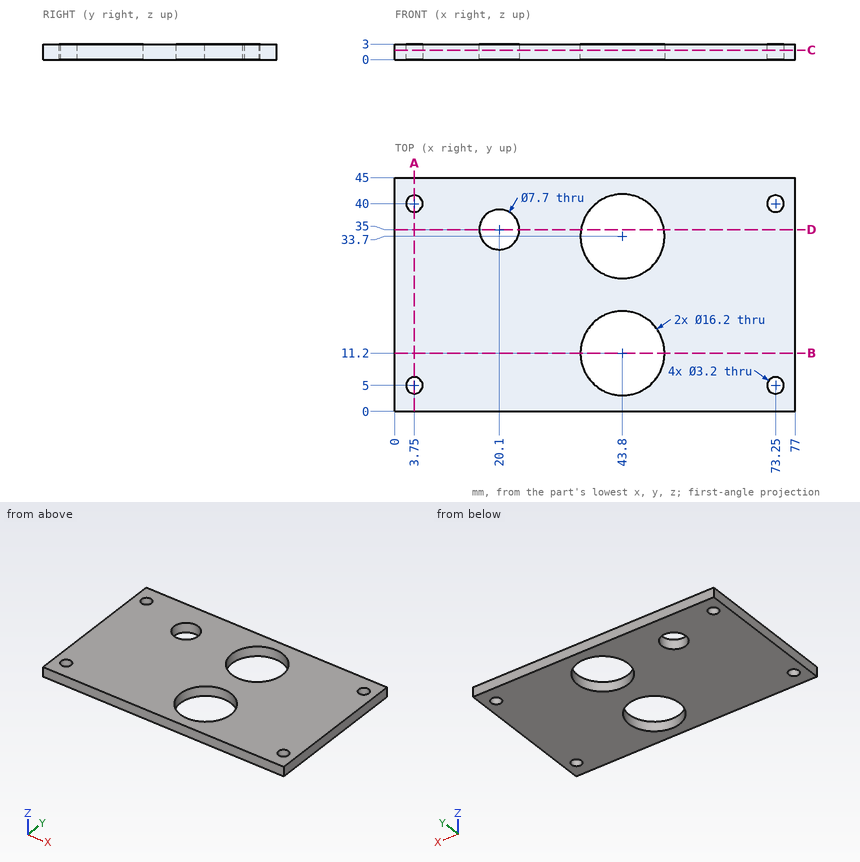
Could you check a few things on this drawing? It's one solid part, dimensions in mm from its lowest x, y, z. Give positions to 0.01 mm unless a question says otherwise; leave off trailing zeros. Order: outer loops, then holes, each group sorted by start corner. A loop starts at its lowest first (then second) coordinate and runs counter-clockwise, first axis right, second up. Notation, with made-up numbers: (46.25, 85.25) -> (93.25, 85.25) arc R24 cw to (93.25, 111.25) -> close; hole circle Ø8 at (-38, 17.25). An arc over 180 degrees is marked (long way). Use CSV: the item, a comma, the result in double quotes. Start each with the question number.
Item 1: I'm going to push a flat-ended pin straight in: P1, Ø1.9, axis at x = 3.75, y = 5, coming from the -Z side. Where does the tip first touch, or does it pass through?
Item 2: Suppose I cut it at A-A (x = 3.75). List the corners of the cut face in (y, z) for me.
Item 3: Suppose I cut it at B-B (y = 11.2). List the corners of the cut face in (x, z) for me, and give its area (3 significant figures).
Item 4: Suppose I cut it at C-C (z = 1.8). List the corners of the cut face in (x, y) for me, and give its area (3 significant figures).
Item 5: If I drill on probe 1 along Y at (x, z) = (43.8, 1.4); probe 2 along Y at (x, z) = (73.25, 2.3); probe 3 along X at (y, z) = (6, 1.5), over which ranges is the centre line in solid material (lowest first)? Write a range as [from, to].
Item 6: Suppose I cut it at D-D (y = 35). List the corners of the cut face in (x, z) for me (3 decimals), and give its area (3 significant figures).
Answer block:
1,P1,"passes through"
2,outline,"(0, 0) -> (3.4, 0) -> (3.4, 3) -> (0, 3) -> close; (6.6, 0) -> (38.4, 0) -> (38.4, 3) -> (6.6, 3) -> close; (41.6, 0) -> (45, 0) -> (45, 3) -> (41.6, 3) -> close"
3,outline,"(0, 0) -> (35.7, 0) -> (35.7, 3) -> (0, 3) -> close; (51.9, 0) -> (77, 0) -> (77, 3) -> (51.9, 3) -> close"
3,area,"182 mm^2"
4,outline,"(0, 0) -> (77, 0) -> (77, 45) -> (0, 45) -> close; hole circle Ø3.2 at (3.75, 5); hole circle Ø3.2 at (3.75, 40); hole circle Ø7.7 at (20.1, 35); hole circle Ø16.2 at (43.8, 11.2); hole circle Ø16.2 at (43.8, 33.7); hole circle Ø3.2 at (73.25, 5); hole circle Ø3.2 at (73.25, 40)"
4,area,"2,970 mm^2"
5,probe 1,"y = [0, 3.1], [19.3, 25.6], [41.8, 45]"
5,probe 2,"y = [0, 3.4], [6.6, 38.4], [41.6, 45]"
5,probe 3,"x = [0, 2.5], [5, 37.59], [50.01, 72], [74.5, 77]"
6,outline,"(0, 0) -> (16.25, 0) -> (16.25, 3) -> (0, 3) -> close; (23.95, 0) -> (35.805, 0) -> (35.805, 3) -> (23.95, 3) -> close; (51.795, 0) -> (77, 0) -> (77, 3) -> (51.795, 3) -> close"
6,area,"160 mm^2"
